```python
from build123d import *

# Parameters (mm, degrees)
F0_R     = 3.571875
F1_DEPTH = 3.175
F2_D     = 6.7564


with BuildPart() as f1:
    # F0 (on Top) → F1 (new body)
    with BuildSketch(Plane.XY):
        with BuildLine():
            Line((7.9375, -1.5875), (7.9375, 9.525))
            Line((7.9375, 9.525), (-7.9375, 9.525))
            Line((-7.9375, 9.525), (-7.9375, -1.5875))
            ThreePointArc((-7.9375, -1.5875), (0, -9.525), (7.9375, -1.5875))
        make_face()
        with Locations((0, -1.5875)):
            Circle(F0_R, mode=Mode.SUBTRACT)
        with Locations((0, -1.5875)):
            Circle(F0_R)
    extrude(amount=-F1_DEPTH)

    # F2 (through all)
    with Locations(Plane.XY):
        with Locations((0, -1.5875)):
            Hole(F2_D / 2)


solid = f1.part
```
Part model, mm, in its own coordinate system. Round coordinates to 2 decimals unless told otherwise and drop trailing zeros. Loops run counter-clockwise (first coordinate to the right, second up) from the corner with the lowest first, then second, coordinate; pieces in that order, holes last. Notation, with made-up numbers: (65.5, 19.5) -> (80.5, 19.5) arc R5 ccw to (80.5, 24.5) -> close; hole circle Ø4 at (8.5, 3.25). An arc over 180 degrees is marked (long way). Use CSV: the item, a comma, the result in double quotes. Start each with the question number.
1) Pull direction Y, two halves, no side cores. Call faces 1 (the flat face through (0, 2, -3.175)), 2 (the cylindrical face through (3.375, -1.439, -1.61)), 3 (the flat face through (0, 9.525, -2)): +Y half, -Y half, draft (parallel to the pull), parting line (faces both ways), or undercut.
2) Cut at D-D, the plane y = -7.75. Write the cut outline in (x, z) (3 decimals), plus the area to 3 significant figures.
3) Cut at C-C, the plane z = -2.45. Write the cut outline in (x, y) (1 decimal), plus the area to 3 significant figures.
4) Cut at B-B, the plane y = -0.25. Write the cut outline in (x, z) (1 decimal), plus the area to 3 significant figures.
5) Wall check: L1, parallel to Y at x = 0, z = -0.65 (3 decimals); L2, parallel to X at y = -4.5, z = -1.9; L3, parallel to X at y = -2, z = -2.7. Give the ranges that are in metal, low to high. Write a range as [from, to].
6) Cut at A-A, the plane x = 0. Write the cut outline in (y, z) (3 decimals).
Determined:
1,face 1,"draft"
1,face 2,"undercut"
1,face 3,"+Y half"
2,outline,"(-5.003, -3.175) -> (5.003, -3.175) -> (5.003, 0) -> (-5.003, 0) -> close"
2,area,"31.8 mm2"
3,outline,"(-7.9, -1.6) arc R7.9 ccw to (7.9, -1.6) -> (7.9, 9.5) -> (-7.9, 9.5) -> close; hole circle Ø6.8 at (0, -1.6)"
3,area,"240 mm2"
4,outline,"(-7.9, -3.2) -> (-3.1, -3.2) -> (-3.1, 0) -> (-7.9, 0) -> close; (3.1, -3.2) -> (7.9, -3.2) -> (7.9, 0) -> (3.1, 0) -> close"
4,area,"30.7 mm2"
5,L1,"y = [-9.525, -4.966], [1.791, 9.525]"
5,L2,"x = [-7.38, -1.71], [1.71, 7.38]"
5,L3,"x = [-7.93, -3.35], [3.35, 7.93]"
6,outline,"(-9.525, -3.175) -> (-4.966, -3.175) -> (-4.966, 0) -> (-9.525, 0) -> close; (1.791, -3.175) -> (9.525, -3.175) -> (9.525, 0) -> (1.791, 0) -> close"
